from build123d import *

# Parameters (mm, degrees)
SKETCH1_R           = 12.5
BOSS_EXTRUDE1_DEPTH = 3
BOSS_EXTRUDE2_START = 3
BOSS_EXTRUDE2_DEPTH = 250
BOSS_EXTRUDE3_START = 243
BOSS_EXTRUDE3_DEPTH = 10


with BuildPart() as part:
    # Sketch1 → Boss-Extrude1 (new body)
    with BuildSketch(Plane(origin=(0, 0, 0), x_dir=(0, 1, 0), z_dir=(0, 0, 1))):
        with BuildLine():
            ThreePointArc((-61.741065417, 0.13908703), (-38.440978301, 32.77013475), (-9.016504978, 60.007603513))
            ThreePointArc((-9.016504978, 60.007603513), (0, 63.02), (9.016504978, 60.007603513))
            ThreePointArc((9.016504978, 60.007603513), (38.440978301, 32.77013475), (61.741065417, 0.13908703))
            ThreePointArc((61.741065417, 0.13908703), (62.284318697, -13.672622652), (51.300957447, -22.064536863))
            ThreePointArc((51.300957447, -22.064536863), (0, -26.52870698), (-51.300957447, -22.064536863))
            ThreePointArc((-51.300957447, -22.064536863), (-62.284318697, -13.672622652), (-61.741065417, 0.13908703))
        make_face()
        with Locations(Location((0, 0, 0), (0, 0, 270))):
            Circle(SKETCH1_R, mode=Mode.SUBTRACT)
    extrude(amount=BOSS_EXTRUDE1_DEPTH)

    # Sketch1<3> → Boss-Extrude2 (add)
    with BuildSketch(Plane(origin=(0, 0, 0), x_dir=(0, 1, 0), z_dir=(0, 0, 1)).offset(BOSS_EXTRUDE2_START)):
        with BuildLine():
            Line((0, 60.02), (0, 63.02))
            ThreePointArc((0, 63.02), (-4.75320667, 62.246982335), (-9.016504978, 60.007603513))
            ThreePointArc((-9.016504978, 60.007603513), (-38.440978301, 32.77013475), (-61.741065417, 0.13908703))
            ThreePointArc((-61.741065417, 0.13908703), (-62.284318697, -13.672622652), (-51.300957447, -22.064536863))
            ThreePointArc((-51.300957447, -22.064536863), (-25.747412733, -25.410559647), (0, -26.52870698))
            Line((0, -26.52870698), (0, -23.52870698))
            ThreePointArc((0, -23.52870698), (-25.487337857, -22.421854065), (-50.782765957, -19.10962949))
            ThreePointArc((-50.782765957, -19.10962949), (-59.569454957, -12.396098122), (-59.134852334, -1.346730376))
            ThreePointArc((-59.134852334, -1.346730376), (-36.189588879, 30.787397836), (-7.213203982, 57.610082811))
            ThreePointArc((-7.213203982, 57.610082811), (-3.802565336, 59.401585868), (0, 60.02))
        make_face()
        with BuildLine():
            ThreePointArc((9.016504978, 60.007603513), (4.75320667, 62.246982335), (0, 63.02))
            Line((0, 63.02), (0, 60.02))
            ThreePointArc((0, 60.02), (3.802565336, 59.401585868), (7.213203982, 57.610082811))
            ThreePointArc((7.213203982, 57.610082811), (36.189588879, 30.787397836), (59.134852334, -1.346730376))
            ThreePointArc((59.134852334, -1.346730376), (59.569454957, -12.396098122), (50.782765957, -19.10962949))
            ThreePointArc((50.782765957, -19.10962949), (25.487337857, -22.421854065), (0, -23.52870698))
            Line((0, -23.52870698), (0, -26.52870698))
            ThreePointArc((0, -26.52870698), (25.747412733, -25.410559647), (51.300957447, -22.064536863))
            ThreePointArc((51.300957447, -22.064536863), (62.284318697, -13.672622652), (61.741065417, 0.13908703))
            ThreePointArc((61.741065417, 0.13908703), (38.440978301, 32.77013475), (9.016504978, 60.007603513))
        make_face()
    extrude(amount=BOSS_EXTRUDE2_DEPTH)

    # Sketch1<4> → Boss-Extrude3 (add)
    with BuildSketch(Plane(origin=(0, 0, 0), x_dir=(0, 1, 0), z_dir=(0, 0, 1)).offset(BOSS_EXTRUDE3_START)):
        with BuildLine():
            Line((0, 63.02), (0, 64.02))
            ThreePointArc((0, 64.02), (-5.070087115, 63.195447824), (-9.617605309, 60.806777081))
            ThreePointArc((-9.617605309, 60.806777081), (-39.191441441, 33.431047055), (-62.609803112, 0.634359498))
            ThreePointArc((-62.609803112, 0.634359498), (-63.189273276, -14.098130829), (-51.473687943, -23.049505987))
            ThreePointArc((-51.473687943, -23.049505987), (-25.834104358, -26.406794841), (0, -27.52870698))
            Line((0, -27.52870698), (0, -26.52870698))
            ThreePointArc((0, -26.52870698), (-25.747412733, -25.410559647), (-51.300957447, -22.064536863))
            ThreePointArc((-51.300957447, -22.064536863), (-62.284318697, -13.672622652), (-61.741065417, 0.13908703))
            ThreePointArc((-61.741065417, 0.13908703), (-38.440978301, 32.77013475), (-9.016504978, 60.007603513))
            ThreePointArc((-9.016504978, 60.007603513), (-4.75320667, 62.246982335), (0, 63.02))
        make_face()
        with BuildLine():
            ThreePointArc((9.617605309, 60.806777081), (5.070087115, 63.195447824), (0, 64.02))
            Line((0, 64.02), (0, 63.02))
            ThreePointArc((0, 63.02), (4.75320667, 62.246982335), (9.016504978, 60.007603513))
            ThreePointArc((9.016504978, 60.007603513), (38.440978301, 32.77013475), (61.741065417, 0.13908703))
            ThreePointArc((61.741065417, 0.13908703), (62.284318697, -13.672622652), (51.300957447, -22.064536863))
            ThreePointArc((51.300957447, -22.064536863), (25.747412733, -25.410559647), (0, -26.52870698))
            Line((0, -26.52870698), (0, -27.52870698))
            ThreePointArc((0, -27.52870698), (25.834104358, -26.406794841), (51.473687943, -23.049505987))
            ThreePointArc((51.473687943, -23.049505987), (63.189273276, -14.098130829), (62.609803112, 0.634359498))
            ThreePointArc((62.609803112, 0.634359498), (39.191441441, 33.431047055), (9.617605309, 60.806777081))
        make_face()
    extrude(amount=BOSS_EXTRUDE3_DEPTH)


solid = part.part
Geometry check sheet. Reference: the model listing, model coordinates, mm. A direction names the side the tool comes from. Give positions to 0.01 mm unless a question says otherwise; leave off trailing zeros. Write each loop counter-clockwise with the first axis right and the second up, starting at its lowest first coordinate (ties: lowest second). Pieces come first, ordered by that corner, then holes. Notation, with made-up numbers: (5.5, -5.75) - (22.5, -5.75) arc R11 cw to (22.5, 2.25) - close; hole circle Ø1 at (62, 82.25). An arc over 180 degrees is marked (long way). Put each result on its own line as item: value.
1. Sectioned sample at C-C, the plane x = 16. Enter the section's corners in (y, z).
Ans:
outline: (-62.13, 243) - (-60.92, 243) - (-60.92, 0) - (60.92, 0) - (60.92, 243) - (62.13, 243) - (62.13, 253) - (56.96, 253) - (56.96, 3) - (-56.96, 3) - (-56.96, 253) - (-62.13, 253) - close
2. Draft check along X on faces 4 (the cylindrical face through (-33.19, -38.07, 119.8)), 5 (the cylindrical face through (14.292, 63.097, 247.93)), 6 (the cylindrical face through (-31, 36, 126)). Enter one of: +X half, -X half, draft (parallel to the pull), parting line (faces both ways), or undercut.
Ans:
face 4: -X half
face 5: parting line
face 6: undercut
3. Sectioned sample at B-B, the plane x = -8. Enter the section's corners in (y, z).
Ans:
outline: (-58.2, 243) - (-57.01, 243) - (-57.01, 0) - (-9.6, 0) - (-9.6, 3) - (-53.45, 3) - (-53.45, 253) - (-58.2, 253) - close; (9.6, 0) - (57.01, 0) - (57.01, 243) - (58.2, 243) - (58.2, 253) - (53.45, 253) - (53.45, 3) - (9.6, 3) - close
4. Thickness scan on line 1 (Z direction, x = -18, y = 28); line 2 (X direction, y = 8, z = 196.5); line 3 (X direction, y = -24, z = 89.5). Record the ranges inside material, lowest first.
Ans:
line 1: z = 0 to 3
line 2: x = -60.71 to -57.02, 23.42 to 26.42
line 3: x = -47.53 to -43.43, 22.55 to 25.56
5. Set-up check for faces 1 (the cylindrical face through (13.85, 62.2, 119.8)), 2 (the cylindrical face through (13.49, -62.37, 119.8)), 3 (the cylindrical face through (12.25, 59.637, 126.25)): record each of +Z, -Z, +X, -X, +Y, -Y from which the full face is reachable in a straight line by a thin tool's end or side.
Ans:
face 1: -Z, +Y
face 2: -Z, -Y
face 3: +Z
6. Go/stop test with flat-tipped pins: pin 1 (3 mm diameter, centred on x = -49, z = 175.5, fed in from +Y); pin 2 (2 mm diameter, centred on y = 45, z = 227.5, fed in from -X); pin 3 (3 mm diameter, centred on y = 17, z = 101, fed in from -X); pin 4 (10 mm diameter, centred on x = -46.5, y = 6.5, fed in from -Z). Record where each tip stops, or that it passes through.
Ans:
pin 1: stops at y = 24.03
pin 2: stops at x = -26.17
pin 3: stops at x = -54.92
pin 4: stops at z = 0
7. Sectioned sample at A-A, the plane z = 60. Enter the section's corners in (x, y), plus the area to 3 significant figures.
Ans:
outline: (-60.01, -9.02) arc R197 ccw to (-0.14, -61.74) arc R15 ccw to (22.06, -51.3) arc R297 ccw to (22.06, 51.3) arc R15 ccw to (-0.14, 61.74) arc R197 ccw to (-60.01, 9.02) arc R15 ccw to start; hole (-57.61, -7.21) arc R194 ccw to (1.35, -59.13) arc R12 ccw to (19.11, -50.78) arc R294 ccw to (19.11, 50.78) arc R12 ccw to (1.35, 59.13) arc R194 ccw to (-57.61, 7.21) arc R12 ccw to start
area: 993 mm²
